from build123d import *


with BuildPart() as part:
    # Sketch1 → Revolve1 (revolve)
    with BuildSketch(Plane.XY):
        with BuildLine():
            Line((508, 25.4), (508, 0))
            Line((508, 0), (482.6, 0))
            Line((482.6, 0), (482.6, 25.4))
            ThreePointArc((482.6, 25.4), (473.944080845, 60.673745801), (449.942857143, 87.933667667))
            ThreePointArc((449.942857143, 87.933667667), (235.791918316, 193.018653743), (0, 229.152435112))
            Line((0, 229.152435112), (0, 254.552435112))
            ThreePointArc((0, 254.552435112), (243.398109229, 217.253047893), (464.457142857, 108.778223555))
            ThreePointArc((464.457142857, 108.778223555), (496.458774459, 72.431661068), (508, 25.4))
        make_face()
    revolve(axis=Axis((0, 254.552435112, 0), (0, -1, 0)))


solid = part.part
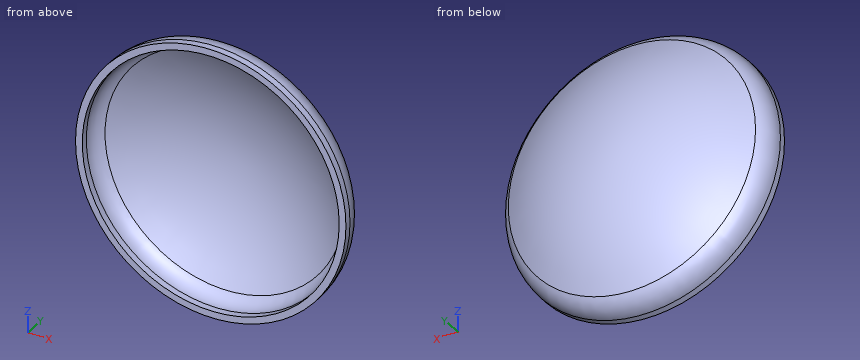
Geometry: final body of the model. Coordinates: model frame, mm. Give positions to 0.01 mm unless a question says otherwise; leave off trailing zeros. Order: outer loops, then holes, each group sorted by start corner. A loop starts at its lowest first (then second) coordinate and runs counter-clockwise, first axis right, second up. Notation, with made-up numbers: (14.25, 37) -> (61.25, 37) arc R20 cw to (61.25, 59) -> close; hole circle Ø3 at (-35, 71.25). An arc over 180 degrees is marked (long way). Answer as a JSON object with one key per item and string values.
Q1. Section C-C (y = 51.5). Output: boundary loops of the cut face in (x, z), plus the area to 3 significant figures.
Entries:
{"outline": "circle Ø1009.18 at (0, 0); hole circle Ø955.98 at (0, 0)", "area": "82,100 mm^2"}
Q2. Section B-B (x = 0). Output: boundary loops of the cut face in (y, z).
Entries:
{"outline": "(0, -508) -> (25.4, -508) arc R101.6 ccw to (108.78, -464.46) arc R812.8 ccw to (108.78, 464.46) arc R101.6 ccw to (25.4, 508) -> (0, 508) -> (0, 482.6) -> (25.4, 482.6) arc R76.2 cw to (87.93, 449.94) arc R787.4 cw to (87.93, -449.94) arc R76.2 cw to (25.4, -482.6) -> (0, -482.6) -> close"}
Q3. Material intervals for probe 1 along Z at (x, y) = (0, 15); probe 2 along X at (y, z) = (58, -294); probe 3 along Z at (x, y) = (-296, 18.5) (3 decimals), sorted ascending.
Entries:
{"probe 1": "z = -508 to -482.6, 482.6 to 508", "probe 2": "x = -407.67 to -373.43, 373.43 to 407.67", "probe 3": "z = -412.853 to -381.165, 381.165 to 412.853"}
Q4. Section A-A (z = 0). Output: boundary loops of the cut face in (x, y).
Entries:
{"outline": "(-508, 0) -> (-482.6, 0) -> (-482.6, 25.4) arc R76.2 cw to (-449.94, 87.93) arc R787.4 cw to (449.94, 87.93) arc R76.2 cw to (482.6, 25.4) -> (482.6, 0) -> (508, 0) -> (508, 25.4) arc R101.6 ccw to (464.46, 108.78) arc R812.8 ccw to (-464.46, 108.78) arc R101.6 ccw to (-508, 25.4) -> close"}
Q5. First-contact query: pin 1 (1 mm diameter, centred on x = -358, z = 279, fed in from -Y); pin 2 (2 mm diameter, centred on x = -99.5, z = -189, fed in from -Y); pin 3 (6 mm diameter, centred on x = 266.5, y = 87, fed in from -Z). Flat tips, straight axial feed; report the tip coordinate or a pass-through.
Entries:
{"pin 1": "stops at y = 84.6", "pin 2": "stops at y = 199.35", "pin 3": "stops at z = -411.13"}
